```python
from build123d import *

# Parameters (mm, degrees)
F1_W           = 57.15
F1_H           = 118.11
F2_DEPTH       = 34.925
F4_D           = 3.81
F4_CBORE_D     = 8.89
F4_CBORE_DEPTH = 12.7


with BuildPart() as f2:
    # F1 (on Front) → F2 (new body, symmetric)
    with BuildSketch(Plane.XZ):
        Rectangle(F1_W, F1_H)
    extrude(amount=F2_DEPTH, both=True)

    # F4 (through all)
    with Locations(Plane.XZ.offset(34.925)):
        with Locations((0, -25.4)):
            CounterBoreHole(F4_D / 2, F4_CBORE_D / 2, F4_CBORE_DEPTH)

    # F5: F2 across plane


with BuildPart() as f2_1:
    add(f2.part)
    add(f2.part.mirror(Plane.XY), mode=Mode.INTERSECT)


solid = f2_1.part
```
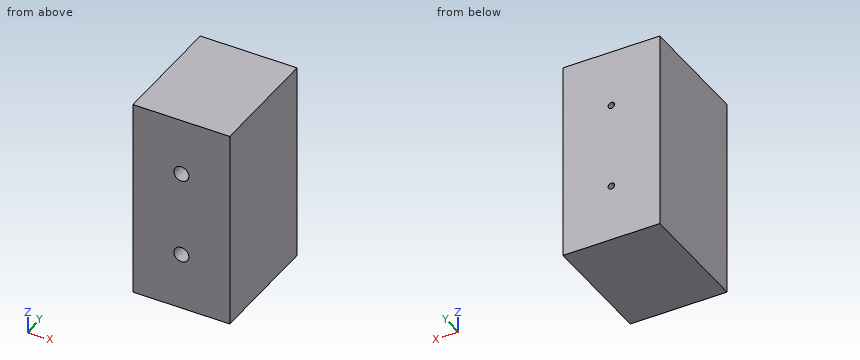
Model file for the job. Use its own axes, mm. Give positions to 0.01 mm unless a question says otherwise; leave off trailing zeros. Loops run counter-clockwise (first coordinate to the right, second up) from the corner with the lowest first, then second, coordinate; pieces in that order, holes last. Notation, with made-up numbers: (81.25, 8.25) -> (139.25, 8.25) arc R8 cw to (139.25, 14.25) -> close; hole circle Ø10 at (35, -10). An arc over 180 degrees is marked (long way). Use CSV: the item, a comma, the result in double quotes. Start each with the question number.
1) Slice it at B-B on x = 0. Give the cut face in (y, z) (3 decimals).
2) Slice it at A-A on z = 25.4. Give the cut face in (x, y) (3 decimals).
3) Flat gauge pins, fed straight in: pin 1 Ø2.5 at (x, z) = (0.5, 26.5) entering from -Y (3 decimals); pin 2 Ø10 at (x, z) = (-0.5, -23.5) entering from -Y (3 decimals). Where does each tip first touch, or does it go through?
4) Wall check: line 1 (Z direction, x = 0, y = -30) (3 decimals); line 2 (X direction, y = -28.75, z = 25.4) (3 decimals); line 3 (X direction, y = -1.5, z = 25.4) (3 decimals). Give the ranges that are in metal, low to high.
Computed values:
1,outline,"(-34.925, -59.055) -> (34.925, -59.055) -> (34.925, -27.305) -> (-22.225, -27.305) -> (-22.225, -29.845) -> (-34.925, -29.845) -> close; (-34.925, -20.955) -> (-22.225, -20.955) -> (-22.225, -23.495) -> (34.925, -23.495) -> (34.925, 23.495) -> (-22.225, 23.495) -> (-22.225, 20.955) -> (-34.925, 20.955) -> close; (-34.925, 29.845) -> (-22.225, 29.845) -> (-22.225, 27.305) -> (34.925, 27.305) -> (34.925, 59.055) -> (-34.925, 59.055) -> close"
2,outline,"(-28.575, -34.925) -> (-4.445, -34.925) -> (-4.445, -22.225) -> (-1.905, -22.225) -> (-1.905, 34.925) -> (-28.575, 34.925) -> close; (1.905, -22.225) -> (4.445, -22.225) -> (4.445, -34.925) -> (28.575, -34.925) -> (28.575, 34.925) -> (1.905, 34.925) -> close"
3,pin 1,"stops at y = -22.225"
3,pin 2,"stops at y = -34.925"
4,line 1,"z = -59.055 to -29.845, -20.955 to 20.955, 29.845 to 59.055"
4,line 2,"x = -28.575 to -4.445, 4.445 to 28.575"
4,line 3,"x = -28.575 to -1.905, 1.905 to 28.575"
